The listing builds one solid part. Answer for the finished solid, in the listing's coordinates (mm). A direction names the side the tool comes from. Give positions to 0.01 mm unless a question says otherwise; leave off trailing zeros. Write each loop counter-clockwise with the first axis right and the second up, starting at its lowest first coordinate (ties: lowest second). Pieces come first, ordered by that corner, then holes. Notation, with made-up numbers: (-22, -38.5) -> (27, -38.5) arc R19 cw to (27, -10.5) -> close; hole circle Ø6 at (80.5, 15). An arc over 180 degrees is marked (long way). One line per question, with ' | ' between items.
from build123d import *

# Parameters (mm, degrees)
F0_W           = 12
F0_H           = 50
F1_DEPTH       = 30
F3_D           = 7
F3_CSINK_D     = 12
F3_CSINK_ANGLE = 90
F4_W           = 4
F4_H           = 17.1277186767
F5_DEPTH       = 50
F11_DEPTH      = 12.5
F12_R          = 2
F15_DEPTH      = 12.5


# Not quite as in the source:
# - two fillets or chamfers of one size are made in one step
# - the dataset's text gives a spline's control points without its knots; the knots are read off the source's solid


with BuildPart() as f1:
    # F0 (on Top) → F1 (new body)
    with BuildSketch(Plane.XY):
        with Locations((0, -25)):
            Rectangle(F0_W, F0_H)
    extrude(amount=F1_DEPTH)

    # F3 (through all)
    with Locations(Plane(origin=(0, 0, 0), x_dir=(1, 0, 0), z_dir=(0, 1, 0))):
        with Locations((0, -10)):
            CounterSinkHole(F3_D / 2, F3_CSINK_D / 2, counter_sink_angle=F3_CSINK_ANGLE)

    # F4 (on Front) → F5 (cut)
    with BuildSketch(Plane.XZ):
        with Locations((0, 21.4361406616)):
            Rectangle(F4_W, F4_H)
    extrude(amount=F5_DEPTH, mode=Mode.SUBTRACT)

    # F10 (on Right) → F11 (cut, symmetric)
    with BuildSketch(Plane.YZ):
        with BuildLine():
            Line((-12.1560385451, 15.6568542495), (0, 15.6568542495))
            Line((0, 15.6568542495), (0, 30))
            Line((0, 30), (-50, 30))
            Line((-50, 30), (-50, 15.0572415441))
            add(Edge.make_bspline(
                [(-10.7545843348, 24.9280158802), (-18.8047000422, 24.9610823092), (-34.6615045914, 23.1331099195), (-44.5054902356, 17.945709156), (-50, 15.0572415441)],
                knots=[0, 0, 0, 0, 0.5383520225, 1, 1, 1, 1], degree=3))
            Line((-10.7545843348, 24.9280158802), (-12.1560385451, 15.6568542495))
        make_face()
    extrude(amount=F11_DEPTH, both=True, mode=Mode.SUBTRACT)

    # F12
    f12_edges = [f1.edges().sort_by_distance(p)[0] for p in [
        (-6, -31.098721, 22.804231),
        (6, -31.098721, 22.804231),
    ]]
    fillet(f12_edges, radius=F12_R)

    # F14 (on Right) → F15 (cut, symmetric)
    with BuildSketch(Plane.YZ):
        Polygon((0, 0), (-50, 5.1978901029), (-50, 0), align=None)
    extrude(amount=F15_DEPTH, both=True, mode=Mode.SUBTRACT)


solid = f1.part
Item 1: Find section A-A (x = 0). Write down the section's boundary in (y, z), then the cut area to 3 significant figures.
Answers below:
outline: (-50, 5.2) -> (0, 0) -> (0, 4) -> (-2.5, 6.5) -> (-50, 6.5) -> close | area: 192 mm²
Item 2: Determine the mould class of faces 1 (the face through (-3.972, -11.446, 20.357)), 2 (the face through (0.084, -24.65, 2.563)), 3 (the face through (3, -50, 7)) for opening direction Z: pulls with the +Z half, pulls with the -Z half, needs draft (parallel to the pull), parting line crosses it, or undercut.
Answers below:
face 1: undercut | face 2: pulls with the -Z half | face 3: needs draft
Item 3: A tool of negligible diameter and unlimited length cuts with its end or side. For faces 4 (the face through (4.028, -11.446, 20.357)), 5 (the face through (2, -25, 17)), 6 (the face through (6, -25, 11)), from which of +Z, -Z, +X, -X, +Y, -Y can it reach the whole face along a straight path? Write none if from no direction.
Answers below:
face 4: +X, -X, +Y | face 5: +Z, +Y, -Y | face 6: +Z, -Z, +X, +Y, -Y
Item 4: Consider line 1 (X direction, y = -32, z = 10); line 2 (X direction, y = -44, z = 13); line 3 (Z direction, x = 3.75, y = -24). Determine where each line is inside the solid, lowest interval first. Write a range as [from, to].
Answers below:
line 1: [-6, -3.5], [3.5, 6] | line 2: [-6, -2], [2, 6] | line 3: [2.49, 24.08]
Item 5: Flat-ended cylindrical pins translate along their axes: pin 1 (1.2 mm diameter, centred on x = -4.5, y = -8, fed in from +Z); pin 2 (3 mm diameter, centred on x = 4.5, y = -35, fed in from +Z). Find the tip coordinate at first contact, or state that the pin passes through.
Answers below:
pin 1: z = 15.66 | pin 2: z = 22.18
